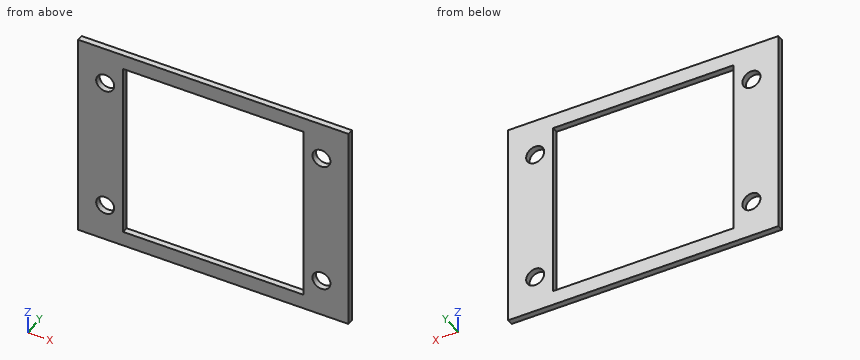
```python
from build123d import *

# Parameters (mm, degrees)
CROQUIS1_R              = 1.5
CROQUIS1_W              = 30
CROQUIS1_H              = 30
SALIENTE_EXTRUIR1_DEPTH = 1
CROQUIS2_W              = 45
CROQUIS2_H              = 5
CORTAR_EXTRUIR1_DEPTH   = 10


with BuildPart() as part:
    # Croquis1 → Saliente-Extruir1 (new body)
    with BuildSketch(Plane(origin=(0, 0, 0), x_dir=(1, 0, 0), z_dir=(0, 1, 0))):
        with BuildLine():
            ThreePointArc((-7.5, -7.398453182), (-7.449747468, -7.449747468), (-7.398453182, -7.5))
            Line((-7.398453182, -7.5), (37.5, -7.5))
            Line((37.5, -7.5), (37.5, 37.5))
            Line((37.5, 37.5), (-7.5, 37.5))
            Line((-7.5, 37.5), (-7.5, -7.398453182))
        make_face()
        with Locations(Location((-3, 3.75, 0), (0, 0, 270))):
            Circle(CROQUIS1_R, mode=Mode.SUBTRACT)
        with Locations(Location((33, 3.75, 0), (0, 0, 270))):
            Circle(CROQUIS1_R, mode=Mode.SUBTRACT)
        with Locations(Location((-3, 26.25, 0), (0, 0, 270))):
            Circle(CROQUIS1_R, mode=Mode.SUBTRACT)
        with Locations((15, 15)):
            Rectangle(CROQUIS1_W, CROQUIS1_H, mode=Mode.SUBTRACT)
        with Locations(Location((33, 26.25, 0), (0, 0, 270))):
            Circle(CROQUIS1_R, mode=Mode.SUBTRACT)
    extrude(amount=SALIENTE_EXTRUIR1_DEPTH)

    # Croquis2 → Cortar-Extruir1 (cut)
    with BuildSketch(Plane(origin=(0, 1, 0), x_dir=(1, 0, 0), z_dir=(0, 1, 0))):
        with Locations((15, 35)):
            Rectangle(CROQUIS2_W, CROQUIS2_H)
        with Locations((15, -5)):
            Rectangle(CROQUIS2_W, CROQUIS2_H)
    extrude(amount=-CORTAR_EXTRUIR1_DEPTH, mode=Mode.SUBTRACT)


solid = part.part
```
Source: CAD feature listing. Evaluate the final solid. Frame: model axes, mm. Give positions to 0.01 mm unless a question says otherwise; leave off trailing zeros. Write each loop counter-clockwise with the first axis right and the second up, starting at its lowest first coordinate (ties: lowest second). Pieces come first, ordered by that corner, then holes.
1. Section query D-D (x = -3). Return the cut outline in (y, z), then the cut area to 3 significant figures.
2. Section query B-B (y = 0.3). Return the cut outline in (x, z).
3. Material intervals for line 1 along X through (y, z) = (0.8, -26.25); line 2 along X through (y, z) = (0.75, -16.5); line 3 along Z through (x, y) = (13.5, 0.3), sorted ascending.
4. Section query A-A (x = 18.5). Return the cut outline in (y, z).
5. Section query C-C (z = -18.5). Return the cut outline in (x, y), then the cut area to 3 significant figures.
Output values:
1. outline: (0, -32.5) - (1, -32.5) - (1, -27.75) - (0, -27.75) - close; (0, -24.75) - (1, -24.75) - (1, -5.25) - (0, -5.25) - close; (0, -2.25) - (1, -2.25) - (1, 2.5) - (0, 2.5) - close
1. area: 29.0 mm2
2. outline: (-7.5, -32.5) - (37.5, -32.5) - (37.5, 2.5) - (-7.5, 2.5) - close; hole circle Ø3 at (-3, -26.25); hole circle Ø3 at (-3, -3.75); hole (0, -30) - (30, -30) - (30, 0) - (0, 0) - close; hole circle Ø3 at (33, -26.25); hole circle Ø3 at (33, -3.75)
3. line 1: x = -7.5 to -4.5, -1.5 to 0, 30 to 31.5, 34.5 to 37.5
3. line 2: x = -7.5 to 0, 30 to 37.5
3. line 3: z = -32.5 to -30, 0 to 2.5
4. outline: (0, -32.5) - (1, -32.5) - (1, -30) - (0, -30) - close; (0, 0) - (1, 0) - (1, 2.5) - (0, 2.5) - close
5. outline: (-7.5, 0) - (0, 0) - (0, 1) - (-7.5, 1) - close; (30, 0) - (37.5, 0) - (37.5, 1) - (30, 1) - close
5. area: 15.0 mm2
